Check sheet for the drawn part. Datum: minimum x, y, z corner. Units: mm. A direction names the side the tool comes from. Coordinates: 2 decimals unless noted, no trailing zeros. Loops run counter-clockwise (first coordinate to the right, second up) from the corner with the lowest first, then second, coordinate; pieces in that order, holes last. Notation, with made-up numbers: (67.25, -15) -> (80.25, -15) arc R5 cw to (80.25, -10) -> close; hole circle Ø3 at (-38.5, 21). An arc over 180 degrees is marked (long way). Use CSV: the item, a comma, the result in double quotes. Start each with the question number.
1. Set-up check for the marked faces 1, 2 and 3: record each of +Z, -Z, +X, -X, +Y, -Y from which the full face is reachable in a straight line by a thin tool's end or side.
2. Sectioned sample at B-B, the plane x = 44. Record the cut outline in (y, z), and give its area (3 significant figures).
3. Thickness scan on L1, parallel to Y at x = 42, z = 7.5; L2, parallel to X at y = 23.5, z = 20; L3, parallel to X at y = 8, z = 20. Record the ranges inside material, lowest first.
4. Sectioned sample at A-A, the plane y = 20.75. Record the cut outline in (x, z) (1 decimal).
5. Gauge pin test, flat ends, axial feed: pin 1 (3 mm diameter, centred on y = 21.5, z = 29, fed in from +X); pin 2 (3 mm diameter, centred on x = 6.5, z = 18, fed in from -Y); pin 3 (1 mm diameter, centred on x = 25.5, y = 13.5, fed in from +Z); pin 4 (2 mm diameter, centred on x = 21.5, z = 14, fed in from +Y). Record the tip position at first contact, or that the pin passes through.
6. Sectioned sample at C-C, the plane x = 51.5. Record the cut outline in (y, z).
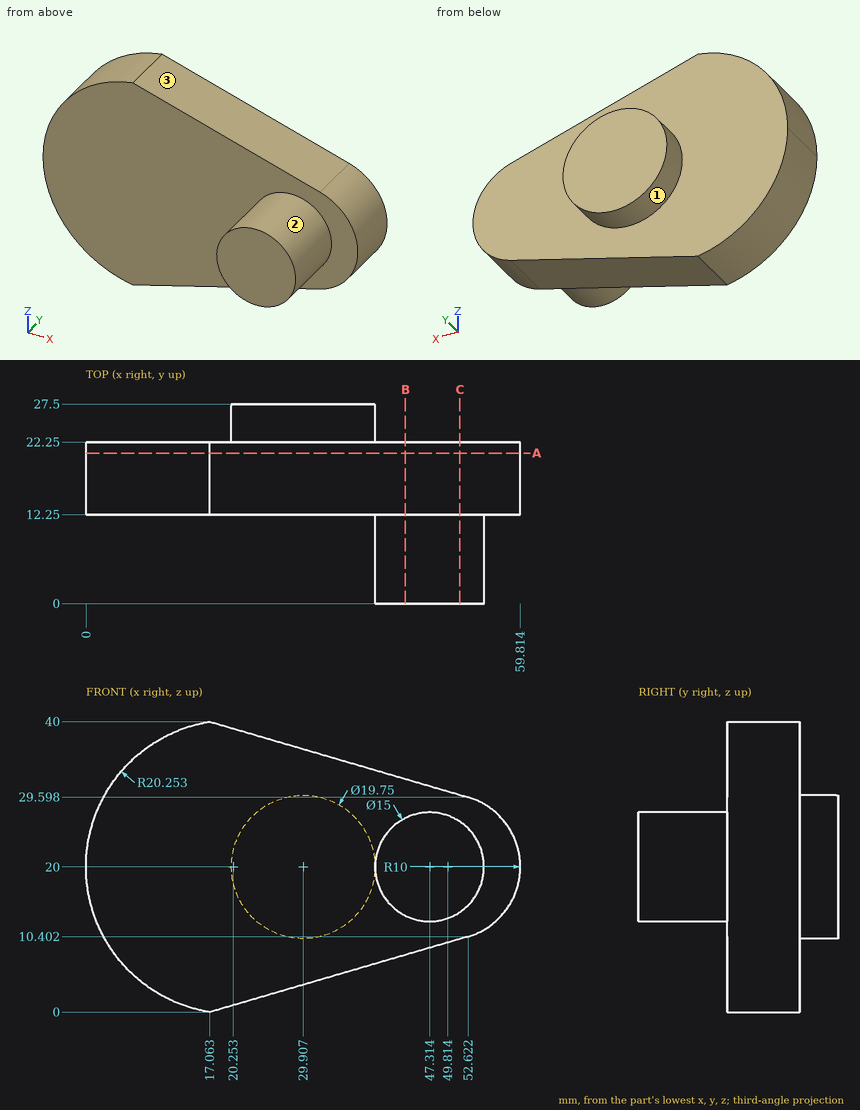
Completed:
1,face 1,"+Y"
1,face 2,"-Y"
1,face 3,"+Z, +X, +Y, -Y"
2,outline,"(0, 13.27) -> (12.25, 13.27) -> (12.25, 7.88) -> (22.25, 7.88) -> (22.25, 32.12) -> (12.25, 32.12) -> (12.25, 26.73) -> (0, 26.73) -> close"
2,area,"407 mm²"
3,L1,"12.25 to 22.25"
3,L2,"20.03 to 39.78"
3,L3,"39.81 to 54.81"
4,outline,"(17.1, 0) -> (52.6, 10.4) arc R10 ccw to (52.6, 29.6) -> (17.1, 40) arc R20.3 ccw to start"
5,pin 1,"x = 56.43"
5,pin 2,"y = 12.25"
5,pin 3,"z = 37.68"
5,pin 4,"y = 27.5"
6,outline,"(0, 13.78) -> (12.25, 13.78) -> (12.25, 10.07) -> (22.25, 10.07) -> (22.25, 29.93) -> (12.25, 29.93) -> (12.25, 26.22) -> (0, 26.22) -> close"
